Work out the finished part from the listing and answer in its coordinate system (mm). Round coordinates to 2 decimals unless told otherwise and drop trailing zeros. Write each loop counter-clockwise with the first axis right and the second up, starting at its lowest first coordinate (ties: lowest second). Pieces come first, ordered by that corner, then holes.
1. Find section B-B (x = 14). Write down the section's boundary in (y, z) (3 decimals).
2. Find section C-C (z = 1.65). Count the separate pieces of the cut face and the enclosed holes in it, and give its area (3 significant figures).
3. Flat-ended cylindrical pins translate along their axes: pin 1 Ø0.9 at (x, z) = (23, 2.5) entering from -Y; pin 2 Ø1 at (y, z) = (-15, 1) entering from +X; pin 3 Ø3 at (x, y) = (3.5, -8) entering from +Z; pin 4 Ø0.9 at (y, z) = (-16, 1) entering from -X. Find the tip coordinate at first contact, or state that the pin passes through.
4. Find section D-D (x = -1). Write down the section's boundary in (y, z) (3 decimals).
5. Find section A-A (y = -2). Write down the section's boundary in (x, z) (3 decimals).
6. Straight lines are drawn through the part: probe 1 along Y at (x, z) = (22, 2.55) (3 decimals); probe 2 along X at (y, z) = (-12, 0.5); probe 3 along X at (y, z) = (2, 0.35). For each, find the intervals that lie inside material, in ascending order.
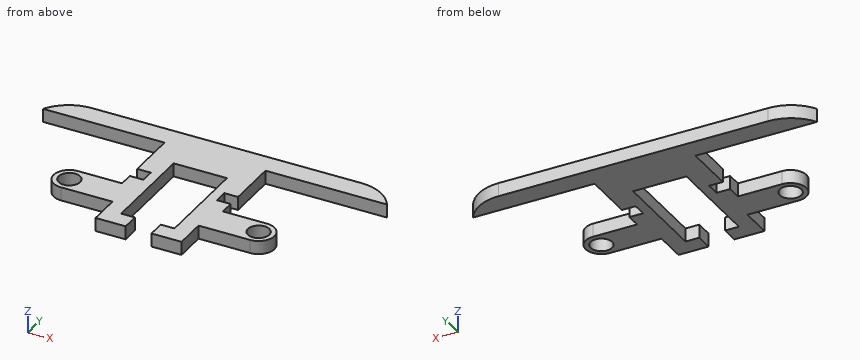
```python
from build123d import *

# Parameters (mm, degrees)
SKETCH1_R           = 2.5
BOSS_EXTRUDE1_DEPTH = 3.125
FILLET1_R           = 10


with BuildPart() as part:
    # Sketch1 → Boss-Extrude1 (new body)
    with BuildSketch(Plane.XY):
        with BuildLine():
            Line((0, 19), (40, 19))
            Line((40, 19), (40, 14))
            Line((40, 14), (11.73, 14))
            Line((11.73, 14), (11.73, 2.17))
            Line((11.73, 2.17), (8.55, 2.17))
            Line((8.55, 2.17), (8.55, -1.01))
            Line((8.55, -1.01), (11.73, -1.01))
            Line((11.73, -1.01), (11.73, -4.34))
            Line((11.73, -4.34), (22, -4.34))
            ThreePointArc((22, -4.34), (25.665, -8.005), (22, -11.67))
            Line((22, -11.67), (10, -11.67))
            Line((10, -11.67), (10, -19))
            Line((10, -19), (3, -19))
            Line((3, -19), (3, -15))
            Line((3, -15), (6.2, -15))
            Line((6.2, -15), (6.2, 7.65))
            Line((6.2, 7.65), (0, 7.65))
            Line((0, 7.65), (0, 19))
        make_face()
        with Locations((22, -8.005)):
            Circle(SKETCH1_R, mode=Mode.SUBTRACT)
    boss_extrude1 = extrude(amount=BOSS_EXTRUDE1_DEPTH)

    # Mirror1: Boss-Extrude1 across plane
    add(boss_extrude1.mirror(Plane(origin=(0, 19, 3.125), x_dir=(0, 0, 1), z_dir=(1, 0, 0))))

    # Fillet1
    # the kernel refuses this fillet: 10 mm, written as the material it takes off along each edge
    with BuildSketch(Plane(origin=(-40, 19, -21.650635095), x_dir=(1, 0, 0), z_dir=(0, 0, 1))) as fillet1_piece_1:
        with BuildLine():
            CenterArc((8.660254038, -10), FILLET1_R, 90, 60)
            Line((0, -5), (-0.173205081, -4.9))
            ThreePointArc((-0.173205081, -4.9), (-0.2, -2.5), (-0.2, 0))
            Line((-0.2, 0), (0, 0.2))
            Line((0, 0.2), (8.660254038, 0.2))
            Line((8.660254038, 0.2), (8.660254038, 0))
        make_face()
    extrude(amount=46.426270189, mode=Mode.SUBTRACT)
    with BuildSketch(Plane(origin=(40, 19, -21.650635095), x_dir=(-1, 0, 0), z_dir=(0, 0, 1))) as fillet1_piece_2:
        with BuildLine():
            CenterArc((8.660254038, 10), FILLET1_R, 210, 60)
            Line((0, 5), (-0.173205081, 4.9))
            ThreePointArc((-0.173205081, 4.9), (-0.2, 2.5), (-0.2, 0))
            Line((-0.2, 0), (0, -0.2))
            Line((0, -0.2), (8.660254038, -0.2))
            Line((8.660254038, -0.2), (8.660254038, 0))
        make_face()
    extrude(amount=46.426270189, mode=Mode.SUBTRACT)


solid = part.part
```
Worked answers:
1. outline: (-11.67, 0) - (-4.34, 0) - (-4.34, 3.125) - (-11.67, 3.125) - close; (14, 0) - (19, 0) - (19, 3.125) - (14, 3.125) - close
2. separate pieces: 1
2. enclosed holes: 2
2. area: 952 mm2
3. pin 1: stops at y = -11.63
3. pin 2: stops at x = 10
3. pin 3: passes through
3. pin 4: stops at x = -10
4. outline: (7.65, 0) - (19, 0) - (19, 3.125) - (7.65, 3.125) - close
5. outline: (-11.73, 0) - (-6.2, 0) - (-6.2, 3.125) - (-11.73, 3.125) - close; (6.2, 0) - (11.73, 0) - (11.73, 3.125) - (6.2, 3.125) - close
6. probe 1: y = -11.67 to -10.505, -5.505 to -4.34, 14 to 19
6. probe 2: x = -10 to -6.2, 6.2 to 10
6. probe 3: x = -8.55 to -6.2, 6.2 to 8.55
